```python
from build123d import *

# Parameters (mm, degrees)
SKETCH1_W           = 185.42
SKETCH1_H           = 241.3
BOSS_EXTRUDE1_DEPTH = 3.175
SKETCH2_R           = 43.815
CUT_EXTRUDE1_DEPTH  = 4.175
SKETCH7_R           = 1.5
CUT_EXTRUDE4_DEPTH  = 4.175
FILLET1_R           = 1.27
SKETCH8_W           = 76.2
SKETCH8_H           = 3.175
CUT_EXTRUDE5_DEPTH  = 4.175
SKETCH11_W          = 3.175
SKETCH11_H          = 76.2
BOSS_EXTRUDE3_DEPTH = 3.175
SKETCH12_W          = 3.302
SKETCH12_H          = 7.874
CUT_EXTRUDE6_DEPTH  = 4.175


with BuildPart() as part:
    # Sketch1 → Boss-Extrude1 (new body)
    with BuildSketch(Plane(origin=(0, 0, 0), x_dir=(1, 0, 0), z_dir=(0, 1, 0))):
        with Locations((92.71, 120.65)):
            Rectangle(SKETCH1_W, SKETCH1_H)
    extrude(amount=BOSS_EXTRUDE1_DEPTH)

    # Sketch2 → Cut-Extrude1 (cut, through all)
    with BuildSketch(Plane(origin=(0, 3.175, 0), x_dir=(1, 0, 0), z_dir=(0, 1, 0))):
        with Locations((145.415, 120.65)):
            Circle(SKETCH2_R)
    extrude(amount=-CUT_EXTRUDE1_DEPTH, mode=Mode.SUBTRACT)

    # Sketch7 → Cut-Extrude4 (cut, through all)
    with BuildSketch(Plane(origin=(0, 3.175, 0), x_dir=(1, 0, 0), z_dir=(0, 1, 0))):
        with Locations((134.62, 171.45)):
            Circle(SKETCH7_R)
        with Locations((134.62, 69.85)):
            Circle(SKETCH7_R)
    extrude(amount=-CUT_EXTRUDE4_DEPTH, mode=Mode.SUBTRACT)

    # Fillet1
    fillet1_edges = [part.edges().sort_by_distance(p)[0] for p in [
        (185.42, 1.5875, -102.779515955),
        (185.42, 1.5875, -138.520484045),
    ]]
    fillet(fillet1_edges, radius=FILLET1_R)

    # Sketch8 → Cut-Extrude5 (cut, through all)
    with BuildSketch(Plane(origin=(0, 3.175, 0), x_dir=(1, 0, 0), z_dir=(0, 1, 0))):
        with Locations((92.71, 239.7125)):
            Rectangle(SKETCH8_W, SKETCH8_H)
        with Locations((92.71, 1.5875)):
            Rectangle(SKETCH8_W, SKETCH8_H)
    extrude(amount=-CUT_EXTRUDE5_DEPTH, mode=Mode.SUBTRACT)

    # Sketch11 → Boss-Extrude3 (add)
    with BuildSketch(Plane(origin=(0, 3.175, 0), x_dir=(1, 0, 0), z_dir=(0, 1, 0))):
        with Locations((-1.5875, 120.65)):
            Rectangle(SKETCH11_W, SKETCH11_H)
    extrude(amount=-BOSS_EXTRUDE3_DEPTH)

    # Sketch12 → Cut-Extrude6 (cut, through all)
    with BuildSketch(Plane(origin=(0, 3.175, 0), x_dir=(1, 0, 0), z_dir=(0, 1, 0))):
        with Locations((175.895, 201.803)):
            Rectangle(SKETCH12_W, SKETCH12_H)
    extrude(amount=-CUT_EXTRUDE6_DEPTH, mode=Mode.SUBTRACT)


solid = part.part
```
Design review of the part built by this model. Coordinates are the model's own, in mm. Give positions to 0.01 mm unless a question says otherwise; leave off trailing zeros. Order: outer loops, then holes, each group sorted by start corner. A loop starts at its lowest first (then second) coordinate and runs counter-clockwise, first axis right, second up. Notation, with made-up numbers: M 56,-30.5 L 98,-30.5 A22 ccw 98,-18.5 Z; hole C 21.25,-1 d6. An arc over 180 degrees is marked long. One line per question, with ' | ' between items. Start each with the question number.
Q1. For pin 1 Ø2.5 at (x, z) = (134.62, -171.45) entering from -Y; pin 2 Ø1.6 at (y, z) = (2, -212) entering from -X, all flat-tipped, find the tip position at first contact; note any pin that passes through.
Q2. For L1, parallel to X at y = 2.4, z = -69.85; L2, parallel to Z at x = 175.5, y = 1.5; L3, parallel to Z at x = 134.62, y = 1, list the stretches that pass through material, from the lowest coordinate up. Write a range as [from, to].
Q3. We need section A-A (x = 160.5). Write out the cut boundary in (y, z) (3 decimals).
Q4. The part is to be moulded in two halves that separate along X. For faces 1 (the face through (90, 0, -122)), 2 (the face through (101.63, 1.61, -122.25)), say which applies: +X half, -X half, draft (parallel to the pull), parting line (faces both ways), or undercut.
Q5. We need section B-B (y = 2.35). Write out the cut boundary in (x, z) (3 decimals), plus the area to 3 significant figures.
Q6. We need section C-C (z = -120.65). Write out the cut boundary in (x, y) (3 decimals), plus the area to 3 significant figures.
Q7. We need section D-D (x = 96.5). Write out the cut boundary in (y, z) (3 decimals).
Returned:
1) pin 1: through | pin 2: x = 0
2) L1: [0, 133.12], [136.12, 185.42] | L2: [-241.3, -205.74], [-197.87, -152.5], [-88.8, 0] | L3: [-241.3, -172.95], [-169.95, -163.11], [-78.19, -71.35], [-68.35, 0]
3) outline: M 0,-241.3 L 3.175,-241.3 L 3.175,-161.786 L 0,-161.786 Z; M 0,-79.514 L 3.175,-79.514 L 3.175,0 L 0,0 Z
4) face 1: draft | face 2: undercut
5) outline: M -3.175,-158.75 L 0,-158.75 L 0,-241.3 L 54.61,-241.3 L 54.61,-238.125 L 130.81,-238.125 L 130.81,-241.3 L 185.42,-241.3 L 185.42,-143.721 A1.27 ccw 183.059,-143.071 A43.815 cw long 183.059,-98.229 A1.27 ccw 185.42,-97.579 L 185.42,0 L 130.81,0 L 130.81,-3.175 L 54.61,-3.175 L 54.61,0 L 0,0 L 0,-82.55 L -3.175,-82.55 Z; hole C 134.62,-171.45 d3; hole C 134.62,-69.85 d3; hole M 174.244,-205.74 L 177.546,-205.74 L 177.546,-197.866 L 174.244,-197.866 Z | area: 38,500 mm2
6) outline: M -3.175,0 L 101.6,0 L 101.6,3.175 L -3.175,3.175 Z | area: 333 mm2
7) outline: M 0,-238.125 L 3.175,-238.125 L 3.175,-3.175 L 0,-3.175 Z
